from build123d import *

# Parameters (mm, degrees)
F0_W     = 25.4
F0_H     = 25.4
F0_R     = 6.35
F1_DEPTH = 76.2
F2_R     = 7.106299
F3_DEPTH = 25.4
F4_SIZE  = 3.175


with BuildPart() as f1:
    # F0 (on Front) → F1 (new body)
    with BuildSketch(Plane.XZ):
        with Locations((-32.064135, 37.379126)):
            Rectangle(F0_W, F0_H)
        with Locations((-32.064135, 37.379126)):
            Circle(F0_R, mode=Mode.SUBTRACT)
    extrude(amount=F1_DEPTH)

    # F2 (on face) → F3 (join)
    with BuildSketch(Plane.XY.offset(50.079126)):
        with Locations((-32.023989, -58.298852)):
            Circle(F2_R)
    extrude(amount=F3_DEPTH)

    # F4
    f4_edges = [f1.edges().sort_by_distance(p)[0] for p in [
        (-19.364135, -38.1, 50.079126),
        (-32.064135, -76.2, 50.079126),
        (-44.764135, -38.1, 50.079126),
        (-32.064135, 0, 50.079126),
    ]]
    chamfer(f4_edges, length=F4_SIZE)


solid = f1.part
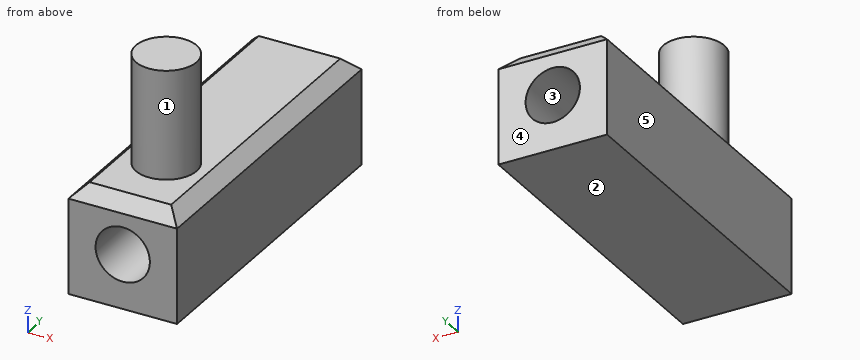
Work out the finished part from the listing and answer in its coordinate system (mm). Face numbers are marked on the shaded views. A direction names the side the tool comes from. Give positions to 0.01 mm unless a question says otherwise; leave off trailing zeros. Loops run counter-clockwise (first coordinate to the right, second up) from the corner with the lowest first, then second, coordinate; pieces in that order, holes last. Notation, with made-up numbers: (-6, 67.25) -> (42, 67.25) arc R26 cw to (42, 86.25) -> close; hole circle Ø11 at (-27.75, 17.5). An arc over 180 degrees is marked (long way). Use a Markdown table: item, result. Add a question column.
1) Which of the six approach directions +Z, -Z, +X, -X, +Y, -Y give full straight-line access (tool end or side, diameter ignored) to the marked faces 1 and 2?
2) The part is cut by section D-D, the plane x = -27. Determine the outline of the cut face in (y, z) (3 decimals), plus the area to 3 significant figures.
3) The part is cut by section B-B, the plane z = 41. Determine the outline of the cut face in (x, y).
4) Each of these flat-tipped pins is pushed along its axis until it touches: P1, Ø4, axis at x = -37.5, y = -43, coming from the +Z side; P2, Ø3, axis at y = -58.5, z = 53.5, coming from the -X side; P3, Ø5, axis at x = -28, z = 56.5, coming from the +Y side. Where does it stop, or does it pass through?
5) Consider line 1 along X through (y, z) = (-21.5, 37); line 2 along Z through (x, y) = (-40.75, -37.5); line 3 along Z through (x, y) = (-29.25, -13). Determine where each line is inside the solid, lowest interval first.
6) The part is cut by section A-A, the plane x = -36. Determine the outline of the cut face in (y, z) (3 decimals).
7) The part is cut by section C-C, the plane y = -61.5. Determine the outline of the cut face in (x, z), plus the area to 3 significant figures.
8) For a pull along X with two mould halves and no side action, classify the marked faces 3, 4 and 5 as +X half, -X half, draft (parallel to the pull), parting line (faces both ways), or undercut.
Reported:
| question | item | result |
|---|---|---|
| 1 | face 1 | +Z |
| 1 | face 2 | -Z, +X, -X, +Y, -Y |
| 2 | outline | (-76.2, 24.679) -> (0, 24.679) -> (0, 33.548) -> (-76.2, 33.548) -> close; (-76.2, 41.21) -> (0, 41.21) -> (0, 46.904) -> (-3.175, 50.079) -> (-53.273, 50.079) -> (-53.273, 75.479) -> (-63.325, 75.479) -> (-63.325, 50.079) -> (-73.025, 50.079) -> (-76.2, 46.904) -> close |
| 2 | area | 1,600 mm^2 |
| 3 | outline | (-44.76, -76.2) -> (-37.28, -76.2) -> (-37.28, 0) -> (-44.76, 0) -> close; (-26.85, -76.2) -> (-19.36, -76.2) -> (-19.36, 0) -> (-26.85, 0) -> close |
| 4 | P1 | stops at z = 50.08 |
| 4 | P2 | stops at x = -39.13 |
| 4 | P3 | stops at y = -51.36 |
| 5 | line 1 | x = -44.76 to -38.4, -25.73 to -19.36 |
| 5 | line 2 | z = 24.68 to 50.08 |
| 5 | line 3 | z = 24.68 to 31.69, 43.07 to 50.08 |
| 6 | outline | (-76.2, 24.679) -> (0, 24.679) -> (0, 32.396) -> (-76.2, 32.396) -> close; (-76.2, 42.362) -> (0, 42.362) -> (0, 46.904) -> (-3.175, 50.079) -> (-52.409, 50.079) -> (-52.409, 75.479) -> (-64.189, 75.479) -> (-64.189, 50.079) -> (-73.025, 50.079) -> (-76.2, 46.904) -> close |
| 7 | outline | (-44.76, 24.68) -> (-19.36, 24.68) -> (-19.36, 46.9) -> (-22.54, 50.08) -> (-25.68, 50.08) -> (-25.68, 75.48) -> (-38.37, 75.48) -> (-38.37, 50.08) -> (-41.59, 50.08) -> (-44.76, 46.9) -> close; hole circle Ø12.7 at (-32.06, 37.38) |
| 7 | area | 831 mm^2 |
| 8 | face 3 | undercut |
| 8 | face 4 | draft |
| 8 | face 5 | -X half |
